Build history of the part. All positions in model axes, mm. Face numbers are marked on the shaded views. Give positions to 0.01 mm unless a question says otherwise; leave off trailing zeros. Write each loop counter-clockwise with the first axis right and the second up, starting at its lowest first coordinate (ties: lowest second). Pieces come first, ordered by that corner, then holes. Notation, with made-up numbers: (7, 24.25) -> (47, 24.25) arc R28 cw to (47, 43.25) -> close; hole circle Ø6 at (61, -24). An arc over 180 degrees is marked (long way). Write item = value, one per line. Start each with the question number.
Q1. Wall check: line 1 (Y direction, x = 2, z = 0); line 2 (Y direction, x = 10.5, z = 0) (3 decimals); line 3 (X direction, y = -58, z = -18.5). Give the ranges that are in metal, low to high.
Q2. Drop flat-ended pins along their axis: P1, Ø8, axis at y = -14, z = 12, coming from the -X side; P2, Ø2, axis at x = 16.5, z = 18.5, coming from the +Y side; P3, Ø1.5, axis at y = -29.5, z = 0, coming from the +X side; P4, Ø10, axis at x = 14, z = -38, coming from the +Y side. Give the stop position or say it passes through.
Q3. Mould opens along Y. For the marked faces 1, 2, 3 and 4 say: pulls with the +Y half, pulls with the -Y half, needs draft (parallel to the pull), parting line crosses it, or undercut.
Q4. Saw through at A-A, the plane y = 0. List the corners of the cut face in (x, z) (3 decimals).
Q5. Saw through at D-D, the plane y = 72.5. List the corners of the cut face in (x, z).
Q6. Saw through at B-B, the plane z = 7.5. List the corners of the cut face in (x, y).
Q7. Saw through at C-C, the plane z = -44. List the corners of the cut face in (x, y), then the cut area to 3 significant figures.
Autodesk Inventor part; units mm, degrees
ref_plane "YZ Plane" through (0, 0, 0) normal (1, 0, 0) x (0, 1, 0)
ref_plane "XZ Plane" through (0, 0, 0) normal (0, 1, 0) x (-1, 0, 0)
ref_plane "XY Plane" through (0, 0, 0) normal (0, 0, 1) x (1, 0, 0)
sketch "Sketch1" plane through (0, 0, 0) normal (1, 0, 0) x (0, 1, 0)
  circle A0 centre (0, -0.3053) radius 87.63
  point P0 (0, 0)
  dimension "d0" = 175.26
extrude "Extrusion1" add sketch "Sketch1" along normal blind 24.638
sketch "Sketch2" plane through (24.638, 0, -0.3053) normal (1, 0, 0) x (0, 0, -1)
  circle A0 centre (-0.3053, 0) radius 84.455
  dimension "d3" = 168.91
extrude "Cut1" cut sketch "Sketch2" against normal blind 21.59
sketch "Sketch3" plane through (3.048, 0, 0) normal (1, 0, 0) x (0, 0, -1)
  circle A0 centre (0, 0) radius 84.455
  circle A1 centre (0, 0) radius 19.05
  dimension "d6" = 38.1
extrude "Cut2" cut sketch "Sketch3" against normal up to next contours A1
equation "\"d7\" = Thickness"
equation "\"BendRadius\" = Thickness"
equation "\"BendReliefWidth\" = Thickness"
equation "\"BendReliefDepth\" = 0.5 * Thickness"
equation "\"CornerReliefSize\" = 4 * Thickness"
equation "\"MinimumRemnant\" = 2 * Thickness"
equation "\"TransitionRadius\" = BendRadius"
equation "\"JacobiRadiusSize\" = BendRadius"
equation "\"GapSize\" = Thickness"
properties part number "Ground_shield_v2" material "Steel, Chrome Plated"
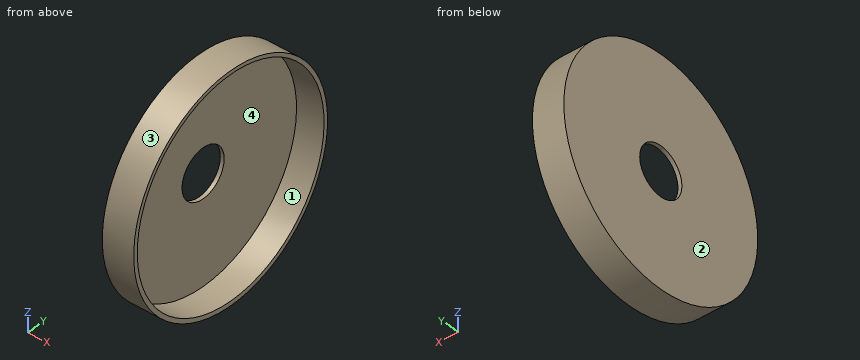
Report:
q1.line_1 = -87.63 to -19.05, 19.05 to 87.63
q1.line_2 = -87.629 to -84.455, 84.455 to 87.629
q1.line_3 = 0 to 3.05
q2.P1 = 0
q2.P2 = 85.8
q2.P3 = 3.05
q2.P4 = 81.3
q3.face_1 = undercut
q3.face_2 = needs draft
q3.face_3 = parting line crosses it
q3.face_4 = undercut
q4.outline = (0, -87.935) -> (24.638, -87.935) -> (24.638, -84.455) -> (3.048, -84.455) -> (3.048, -19.05) -> (0, -19.05) -> close; (0, 19.05) -> (3.048, 19.05) -> (3.048, 84.455) -> (24.638, 84.455) -> (24.638, 87.325) -> (0, 87.325) -> close
q5.outline = (0, -49.53) -> (24.64, -49.53) -> (24.64, -43.32) -> (3.05, -43.32) -> (3.05, 43.32) -> (24.64, 43.32) -> (24.64, 48.92) -> (0, 48.92) -> close
q6.outline = (0, -87.28) -> (24.64, -87.28) -> (24.64, -84.12) -> (3.05, -84.12) -> (3.05, -17.51) -> (0, -17.51) -> close; (0, 17.51) -> (3.05, 17.51) -> (3.05, 84.12) -> (24.64, 84.12) -> (24.64, 87.28) -> (0, 87.28) -> close
q7.outline = (0, -75.96) -> (24.64, -75.96) -> (24.64, -72.09) -> (3.05, -72.09) -> (3.05, 72.09) -> (24.64, 72.09) -> (24.64, 75.96) -> (0, 75.96) -> close
q7.area = 630 mm2
